from build123d import *

# Parameters (mm, degrees)
BOSS_EXTRUDE1_DEPTH = 2.54
SKETCH2_W           = 12.7
SKETCH2_H           = 5.08
BOSS_EXTRUDE2_DEPTH = 12.7
CUT_EXTRUDE2_DEPTH  = 101.731669178
SKETCH4_R           = 1.905
CUT_EXTRUDE3_DEPTH  = 101.731669178
SKETCH5_R           = 1.27
CUT_EXTRUDE4_DEPTH  = 105.216075999
FILLET2_R           = 2.54


with BuildPart() as part:
    # Sketch1 → Boss-Extrude1 (new body)
    with BuildSketch(Plane.XY):
        with BuildLine():
            Line((73.161588965, -6.18197174), (88.401588965, -6.18197174))
            ThreePointArc((88.401588965, -6.18197174), (91.993691413, -7.669869292), (93.481588965, -11.26197174))
            Line((93.481588965, -11.26197174), (93.481588965, -39.20197174))
            ThreePointArc((93.481588965, -39.20197174), (91.993691413, -42.794074189), (88.401588965, -44.28197174))
            Line((88.401588965, -44.28197174), (73.161588965, -44.28197174))
            ThreePointArc((73.161588965, -44.28197174), (69.569486517, -42.794074189), (68.081588965, -39.20197174))
            Line((68.081588965, -39.20197174), (68.081588965, -11.26197174))
            ThreePointArc((68.081588965, -11.26197174), (69.569486517, -7.669869292), (73.161588965, -6.18197174))
        make_face()
    extrude(amount=BOSS_EXTRUDE1_DEPTH)

    # Sketch2 → Boss-Extrude2 (add)
    with BuildSketch(Plane.XY.offset(2.54)):
        with Locations((80.781588965, -12.53197174)):
            Rectangle(SKETCH2_W, SKETCH2_H)
        with Locations((80.781588965, -37.93197174)):
            Rectangle(SKETCH2_W, SKETCH2_H)
    extrude(amount=BOSS_EXTRUDE2_DEPTH)

    # Sketch3 → Cut-Extrude2 (cut, through all)
    with BuildSketch(Plane(origin=(0, -40.47197174, 0), x_dir=(-1, 0, 0), z_dir=(0, -1, 0))):
        with BuildLine():
            Line((-74.431588965, -15.24), (-74.431588965, -8.89))
            ThreePointArc((-74.431588965, -8.89), (-76.291460904, -13.380128061), (-80.781588965, -15.24))
            Line((-80.781588965, -15.24), (-74.431588965, -15.24))
        make_face()
        with BuildLine():
            Line((-87.131588965, -15.24), (-80.781588965, -15.24))
            ThreePointArc((-80.781588965, -15.24), (-85.271717026, -13.380128061), (-87.131588965, -8.89))
            Line((-87.131588965, -8.89), (-87.131588965, -15.24))
        make_face()
    extrude(amount=-CUT_EXTRUDE2_DEPTH, mode=Mode.SUBTRACT)

    # Sketch4 → Cut-Extrude3 (cut, through all)
    with BuildSketch(Plane.XZ.offset(40.47197174)):
        with Locations((80.781588965, 8.89)):
            Circle(SKETCH4_R)
    extrude(amount=-CUT_EXTRUDE3_DEPTH, mode=Mode.SUBTRACT)

    # Sketch5 → Cut-Extrude4 (cut, through all)
    with BuildSketch(Plane.XY.offset(2.54)):
        with Locations((80.781588965, -18.88197174)):
            Circle(SKETCH5_R)
        with BuildLine():
            Line((79.511588965, -32.53447174), (79.511588965, -30.62947174))
            ThreePointArc((79.511588965, -30.62947174), (80.781588965, -29.35947174), (82.051588965, -30.62947174))
            Line((82.051588965, -30.62947174), (82.051588965, -32.53447174))
            ThreePointArc((82.051588965, -32.53447174), (80.781588965, -33.80447174), (79.511588965, -32.53447174))
        make_face()
    extrude(amount=-CUT_EXTRUDE4_DEPTH, mode=Mode.SUBTRACT)

    # Fillet2
    fillet2_edges = [part.edges().sort_by_distance(p)[0] for p in [
        (74.431588965, -12.53197174, 2.54),
        (87.131588965, -12.53197174, 2.54),
        (87.131588965, -37.93197174, 2.54),
        (74.431588965, -37.93197174, 2.54),
    ]]
    fillet(fillet2_edges, radius=FILLET2_R)


solid = part.part
For this review, take the finished solid that the model builds, in its own axes (mm). A direction names the side the tool comes from. Give positions to 0.01 mm unless a question says otherwise; leave off trailing zeros. Order: outer loops, then holes, each group sorted by start corner. A loop starts at its lowest first (then second) coordinate and runs counter-clockwise, first axis right, second up. Notation, with made-up numbers: M -11,57.5 L 36,57.5 A27 ccw 36,91.5 Z; hole C 75.5,1.25 d8. An arc over 180 degrees is marked long. Answer in a Markdown table with one row per item. Add a question column.
(1) For faces 1 (the face through (79.512, -32, 1)), 2 (the face through (68.082, -25, 1)), 3 (the face through (79, -35.392, 7)), 4 (the face through (74.432, -38, 7)), list the 3-axis set-ups (+Z, -Z, +X, -X, +Y, -Y) from which the entire face can be reached by the end or side of a thin tool; tool diameter is ignored.
(2) Consider section B-B on y = -36. State the section outline as (x, z) points (3 decimals), and give its area (3 significant figures).
(3) Wall thickness on probe 1 along Y at (x, z) = (83.75, 8.75); probe 2 along Z at (x, y) = (80.75, -11.5); probe 3 along Z at (x, y) = (85, -34): over which ranges is each line inside the solid? List them lowest first. Write a range as [from, to].
(4) Consider section A-A on z = 5.5. State the section outline as (x, y) points.
(5) Mouldability with a two-part tool opening along Y and no side actions: class faces 5 (the face through (80.81, -33.804, 1.288)), 6 (the face through (81, -6.182, 1)), 7 (the face through (87.132, -38, 7)) as +Y half, -Y half, draft (parallel to the pull), parting line (faces both ways), or undercut.
(6) For pin 1 (3 mm diameter, centred on y = -37, z = 7.5, fed in from -X); pin 2 (4.5 mm diameter, centred on x = 80.78, z = 8.89, fed in from +Y); pin 3 (7.5 mm diameter, centred on x = 86.5, y = -17, fed in from +Z); pin 4 (2 mm diameter, centred on x = 89.5, z = 8, fed in from +Y) (1 decimal), all flat-tipped, find the tip position at first contact; note any pin that passes through.
(7) Consider section C-C on y = -31.5. State the section outline as (x, z) points, and give its area (3 significant figures).
(8) Consider section D-D on z = 9.5. State the section outline as (x, y) points, and give its area (3 significant figures).
Evaluation:
| question | item | result |
|---|---|---|
| 1 | face 1 | +Z, -Z |
| 1 | face 2 | +Z, -Z, -X, +Y, -Y |
| 1 | face 3 | +Z, +X, -X |
| 1 | face 4 | +Z, -X, +Y, -Y |
| 2 | outline | M 68.082,0 L 93.482,0 L 93.482,2.54 L 89.672,2.54 A2.54 cw 87.132,5.08 L 87.132,8.89 A6.35 ccw 74.432,8.89 L 74.432,5.08 A2.54 cw 71.892,2.54 L 68.082,2.54 Z; hole C 80.782,8.89 d3.81 |
| 2 | area | 200 mm^2 |
| 3 | probe 1 | y = [-40.47, -35.39], [-15.07, -9.99] |
| 3 | probe 2 | z = [0, 6.99], [10.79, 15.24] |
| 3 | probe 3 | z = [0, 2.54] |
| 4 | outline | M 74.43,-40.47 L 87.13,-40.47 L 87.13,-35.39 L 74.43,-35.39 Z; M 74.43,-15.07 L 87.13,-15.07 L 87.13,-9.99 L 74.43,-9.99 Z |
| 5 | face 5 | undercut |
| 5 | face 6 | +Y half |
| 5 | face 7 | draft |
| 6 | pin 1 | stops at x = 74.43 |
| 6 | pin 2 | stops at y = -9.99 |
| 6 | pin 3 | stops at z = 14.73 |
| 6 | pin 4 | passes through |
| 7 | outline | M 68.08,0 L 79.51,0 L 79.51,2.54 L 68.08,2.54 Z; M 82.05,0 L 93.48,0 L 93.48,2.54 L 82.05,2.54 Z |
| 7 | area | 58.1 mm^2 |
| 8 | outline | M 74.46,-40.47 L 78.98,-40.47 L 78.98,-35.39 L 74.46,-35.39 Z; M 74.46,-15.07 L 78.98,-15.07 L 78.98,-9.99 L 74.46,-9.99 Z; M 82.59,-40.47 L 87.1,-40.47 L 87.1,-35.39 L 82.59,-35.39 Z; M 82.59,-15.07 L 87.1,-15.07 L 87.1,-9.99 L 82.59,-9.99 Z |
| 8 | area | 91.8 mm^2 |
